```python
from build123d import *

# Parameters (mm, degrees)
SKETCH1_W               = 250
SKETCH1_H               = 50
BOSS_EXTRUDE1_DEPTH     = 55
CUT_EXTRUDE2_DEPTH      = 146.430395722
CUT_EXTRUDE2_DEPTH_BACK = 146.430395722
SKETCH4_OUTSIDE_W       = 304.164
SKETCH4_OUTSIDE_H       = 109.164
FILLET2_R               = 2
CUT_EXTRUDE3_DEPTH      = 143.762915509
CUT_EXTRUDE3_DEPTH_BACK = 143.762915509
SKETCH7_R               = 2.5
SKETCH12_W              = 86.46924187
SKETCH12_H              = 64.710234819
CUT_EXTRUDE7_DEPTH      = 10
CUT_EXTRUDE8_DEPTH      = 10
SKETCH14_R              = 2.5
BOSS_EXTRUDE2_DEPTH     = 30
SKETCH16_W              = 96.26246385
SKETCH16_H              = 15
CUT_EXTRUDE9_DEPTH      = 50
FILLET3_R               = 4.2
FILLET4_R               = 23


with BuildPart() as part:
    # Sketch1 → Boss-Extrude1 (new body)
    with BuildSketch(Plane(origin=(0, 0, 0), x_dir=(1, 0, 0), z_dir=(0, 1, 0))):
        Rectangle(SKETCH1_W, SKETCH1_H)
    extrude(amount=BOSS_EXTRUDE1_DEPTH)

    # Sketch4 outside → Cut-Extrude2 (cut, two sides: drawn at the far end of the back side and taken through both)
    with BuildSketch(Plane.XY.offset(25).offset(-CUT_EXTRUDE2_DEPTH_BACK)):
        with Locations((0, 27.5)):
            Rectangle(SKETCH4_OUTSIDE_W, SKETCH4_OUTSIDE_H)
        with BuildLine():
            Line((-72.5, 42.5), (-72.5, 12.5))
            ThreePointArc((-72.5, 12.5), (16.389156704, 14.940062989), (105, 7.5))
            ThreePointArc((105, 7.5), (125, 27.5), (105, 47.5))
            ThreePointArc((105, 47.5), (16.389156704, 40.059937011), (-72.5, 42.5))
        make_face(mode=Mode.SUBTRACT)
    extrude(amount=CUT_EXTRUDE2_DEPTH + CUT_EXTRUDE2_DEPTH_BACK, mode=Mode.SUBTRACT)

    # Fillet2
    fillet2_edges = [part.edges().sort_by_distance(p)[0] for p in [
        (16.389156704, 14.940062989, 25),
        (16.389156704, 40.059937011, 25),
        (16.389156704, 40.059937011, -25),
        (16.389156704, 14.940062989, -25),
    ]]
    fillet(fillet2_edges, radius=FILLET2_R)

    # Sketch7 → Cut-Extrude3 (cut, two sides: drawn at the far end of the back side and taken through both)
    with BuildSketch(Plane.XY.offset(25).offset(-CUT_EXTRUDE3_DEPTH_BACK)):
        with Locations((105, 27.5)):
            Circle(SKETCH7_R)
    extrude(amount=CUT_EXTRUDE3_DEPTH + CUT_EXTRUDE3_DEPTH_BACK, mode=Mode.SUBTRACT)

    # Sketch12 → Cut-Extrude7 (cut)
    with BuildSketch(Plane.XY.offset(25)):
        with Locations((108.234620935, 27.636294559)):
            Rectangle(SKETCH12_W, SKETCH12_H)
    extrude(amount=-CUT_EXTRUDE7_DEPTH, mode=Mode.SUBTRACT)

    # Sketch13 → Cut-Extrude8 (cut)
    with BuildSketch(Plane(origin=(0, 0, -25), x_dir=(-1, 0, 0), z_dir=(0, 0, -1))):
        with BuildLine():
            Line((-65, 42.911811435), (-65, 12.088188565))
            ThreePointArc((-65, 12.088188565), (-85.028868782, 10.045773403), (-105, 7.5))
            ThreePointArc((-105, 7.5), (-125, 27.5), (-105, 47.5))
            ThreePointArc((-105, 47.5), (-85.028868782, 44.954226597), (-65, 42.911811435))
        make_face()
    extrude(amount=-CUT_EXTRUDE8_DEPTH, mode=Mode.SUBTRACT)

    # Sketch14 → Boss-Extrude2 (add)
    # profile 1 of 2: a face of its own
    with BuildSketch(Plane(origin=(0, 42.5, 0), x_dir=(0, 0, 1), z_dir=(0, -1, 0))):
        with BuildLine():
            Line((-8.002367609, 72.5), (-12.669393759, 94.084995944))
            ThreePointArc((-12.669393759, 94.084995944), (-21.584995944, 99.830606241), (-27.330606241, 90.915004056))
            Line((-27.330606241, 90.915004056), (-23.348983742, 72.5))
            Line((-23.348983742, 72.5), (-8.002367609, 72.5))
        make_face()
        with Locations(Location((-20, 92.5, 0), (0, 0, 180))):
            Circle(SKETCH14_R, mode=Mode.SUBTRACT)
    # profile 2 of 2: a face of its own
    with BuildSketch(Plane(origin=(0, 42.5, 0), x_dir=(0, 0, 1), z_dir=(0, -1, 0))):
        with BuildLine():
            Line((27.330606241, 90.915004056), (23.348983742, 72.5))
            Line((23.348983742, 72.5), (8.002367609, 72.5))
            Line((8.002367609, 72.5), (12.669393759, 94.084995944))
            ThreePointArc((12.669393759, 94.084995944), (21.584995944, 99.830606241), (27.330606241, 90.915004056))
        make_face()
        with Locations((20, 92.5)):
            Circle(SKETCH14_R, mode=Mode.SUBTRACT)
    extrude(amount=BOSS_EXTRUDE2_DEPTH)

    # Sketch16 → Cut-Extrude9 (cut)
    with BuildSketch(Plane.ZY.offset(72.5)):
        with Locations((4.383084191, 27.5)):
            Rectangle(SKETCH16_W, SKETCH16_H)
    extrude(amount=CUT_EXTRUDE9_DEPTH, mode=Mode.SUBTRACT)

    # Fillet3
    fillet3_edges = [part.edges().sort_by_distance(p)[0] for p in [
        (-72.5, 16.25, -8.002367609),
        (-72.5, 16.25, 8.002367609),
        (-72.5, 38.75, 8.002367609),
        (-72.5, 38.75, -8.002367609),
    ]]
    fillet(fillet3_edges, radius=FILLET3_R)

    # Fillet4
    # the kernel refuses this fillet: 23 mm, written as the material it adds along each edge
    with BuildSketch(Plane(origin=(-72.5, 42.030514973, -23.348983742), x_dir=(0, 0, -1), z_dir=(0, -1, 0))) as fillet4_piece_1_section:
        with BuildLine():
            CenterArc((24.342833905, -3.752520734), FILLET4_R, 170.610040363, 21.590428365)
            Line((1.8623081, -8.613174962), (0, 0))
            Line((0, 0), (1.651016258, 0))
        make_face()
    fillet4_piece_1 = extrude(amount=51.530241063, mode=Mode.PRIVATE)
    fillet4_piece_1 = split(fillet4_piece_1, bisect_by=Plane(origin=(-72.5, 35, -23.348983742), z_dir=(0, 1, 0)), keep=Keep.TOP, mode=Mode.PRIVATE)
    add(fillet4_piece_1)
    with BuildSketch(Plane(origin=(-72.5, 20, -23.348983742), x_dir=(0, 0, -1), z_dir=(0, -1, 0))) as fillet4_piece_2_section:
        with BuildLine():
            CenterArc((24.342833905, -3.752520734), FILLET4_R, 170.610040363, 21.590428365)
            Line((1.8623081, -8.613174962), (0, 0))
            Line((0, 0), (1.651016258, 0))
        make_face()
    fillet4_piece_2 = extrude(amount=29.49972609, mode=Mode.PRIVATE)
    fillet4_piece_2 = split(fillet4_piece_2, bisect_by=Plane(origin=(-72.5, 12.5, -23.348983742), z_dir=(0, 1, 0)), keep=Keep.TOP, mode=Mode.PRIVATE)
    add(fillet4_piece_2)
    with BuildSketch(Plane(origin=(-72.5, 64.49972609, -23.348983742), x_dir=(0, 0, -1), z_dir=(0, -1, 0))) as fillet4_piece_3_section:
        with BuildLine():
            CenterArc((24.342833905, -3.752520734), FILLET4_R, 170.610040363, 21.590428365)
            Line((1.8623081, -8.613174962), (0, 0))
            Line((0, 0), (1.651016258, 0))
        make_face()
    fillet4_piece_3 = extrude(amount=29.49972609, mode=Mode.PRIVATE)
    fillet4_piece_3 = split(fillet4_piece_3, bisect_by=Plane(origin=(-72.5, 42.5, -23.348983742), z_dir=(0, -1, 0)), keep=Keep.TOP, mode=Mode.PRIVATE)
    add(fillet4_piece_3)
    with BuildSketch(Plane(origin=(-72.5, 64.49972609, -23.348983742), x_dir=(0, 0, -1), z_dir=(0, -1, 0))) as fillet4_piece_4_section:
        with BuildLine():
            CenterArc((24.342833905, -3.752520734), FILLET4_R, 170.610040363, 21.590428365)
            Line((1.8623081, -8.613174962), (0, 0))
            Line((0, 0), (1.651016258, 0))
        make_face()
    fillet4_piece_4 = extrude(amount=51.530241063, mode=Mode.PRIVATE)
    fillet4_piece_4 = split(fillet4_piece_4, bisect_by=Plane(origin=(-72.5, 20, -23.348983742), z_dir=(0, -1, 0)), keep=Keep.TOP, mode=Mode.PRIVATE)
    add(fillet4_piece_4)
    with BuildSketch(Plane(origin=(-72.5, 42.030514973, 23.348983742), x_dir=(0, 0, 1), z_dir=(0, -1, 0))) as fillet4_piece_5_section:
        with BuildLine():
            CenterArc((24.342833905, 3.752520734), FILLET4_R, 167.799531273, 21.590428365)
            Line((1.8623081, 8.613174962), (0, 0))
            Line((0, 0), (1.651016258, 0))
        make_face()
    fillet4_piece_5 = extrude(amount=51.530241063, mode=Mode.PRIVATE)
    fillet4_piece_5 = split(fillet4_piece_5, bisect_by=Plane(origin=(-72.5, 35, 23.348983742), z_dir=(0, 1, 0)), keep=Keep.TOP, mode=Mode.PRIVATE)
    add(fillet4_piece_5)
    with BuildSketch(Plane(origin=(-72.5, 20, 23.348983742), x_dir=(0, 0, 1), z_dir=(0, -1, 0))) as fillet4_piece_6_section:
        with BuildLine():
            CenterArc((24.342833905, 3.752520734), FILLET4_R, 167.799531273, 21.590428365)
            Line((1.8623081, 8.613174962), (0, 0))
            Line((0, 0), (1.651016258, 0))
        make_face()
    fillet4_piece_6 = extrude(amount=29.49972609, mode=Mode.PRIVATE)
    fillet4_piece_6 = split(fillet4_piece_6, bisect_by=Plane(origin=(-72.5, 12.5, 23.348983742), z_dir=(0, 1, 0)), keep=Keep.TOP, mode=Mode.PRIVATE)
    add(fillet4_piece_6)
    with BuildSketch(Plane(origin=(-72.5, 64.49972609, 23.348983742), x_dir=(0, 0, 1), z_dir=(0, -1, 0))) as fillet4_piece_7_section:
        with BuildLine():
            CenterArc((24.342833905, 3.752520734), FILLET4_R, 167.799531273, 21.590428365)
            Line((1.8623081, 8.613174962), (0, 0))
            Line((0, 0), (1.651016258, 0))
        make_face()
    fillet4_piece_7 = extrude(amount=29.49972609, mode=Mode.PRIVATE)
    fillet4_piece_7 = split(fillet4_piece_7, bisect_by=Plane(origin=(-72.5, 42.5, 23.348983742), z_dir=(0, -1, 0)), keep=Keep.TOP, mode=Mode.PRIVATE)
    add(fillet4_piece_7)
    with BuildSketch(Plane(origin=(-72.5, 64.49972609, 23.348983742), x_dir=(0, 0, 1), z_dir=(0, -1, 0))) as fillet4_piece_8_section:
        with BuildLine():
            CenterArc((24.342833905, 3.752520734), FILLET4_R, 167.799531273, 21.590428365)
            Line((1.8623081, 8.613174962), (0, 0))
            Line((0, 0), (1.651016258, 0))
        make_face()
    fillet4_piece_8 = extrude(amount=51.530241063, mode=Mode.PRIVATE)
    fillet4_piece_8 = split(fillet4_piece_8, bisect_by=Plane(origin=(-72.5, 20, 23.348983742), z_dir=(0, -1, 0)), keep=Keep.TOP, mode=Mode.PRIVATE)
    add(fillet4_piece_8)


solid = part.part
```
For this review, take the finished solid that the model builds, in its own axes (mm). A direction names the side the tool comes from. Coordinates: 2 decimals unless noted, no trailing zeros. Loops run counter-clockwise (first coordinate to the right, second up) from the corner with the lowest first, then second, coordinate; pieces in that order, holes last.
1. For faces 5 (the flat face through (-86, 42.5, 19)), 6 (the flat face through (-84.821, 38.802, 10.666)), 7 (the flat face through (-5, 27, -25)), list the 3-axis set-ups (+Z, -Z, +X, -X, +Y, -Y) from which the entire face can be reached by the end or side of a thin tool; tool diameter is ignored.
2. Add section B-B, the plane y = 27.5. Give the boundary of the cut face in (x, z).
3. For line 1 (X direction, y = 15.75, z = -20); line 2 (Z direction, x = -92, y = 18); line 3 (Y direction, x = 105, z = -8), list the stretches that pass through material, from the lowest coordinate up.
4. Mouldability with a two-part tool opening along Y and no side actions: class faces 1 (the flat face through (-72.5, 28, 0)), 2 (the flat face through (-86, 35, -19)), 3 (the flat face through (-86.083, 16.303, 26.286)), 4 (the flat face through (-86, 12.5, -19)) as +Y half, -Y half, draft (parallel to the pull), parting line (faces both ways), or undercut.
5. Insertion check: P1, Ø8, axis at y = 22, z = 21.5, coming from the +X side; P2, Ø4, axis at x = -35.5, y = 36.5, coming from the +Z side; P3, Ø12, axis at x = 69, z = 1.5, coming from the +Y side. Each pin has a flat end and moves straight along its axis. Give the tip position at first contact, or say it passes through.
6. Add section A-A, the plane z = -20. Give the boundary of the cut face in (x, y), then the cut area to 3 significant figures.
Result:
1. face 5: +Z, -Z, -X, +Y
1. face 6: -X, +Y, -Y
1. face 7: -Z, +X, +Y, -Y
2. outline: (-72.5, -25) - (65, -25) - (65, -15) - (102.5, -15) - (102.5, 15) - (65, 15) - (65, 25) - (-72.5, 25) - close; (107.5, -15) - (125, -15) - (125, 15) - (107.5, 15) - close
3. line 1: x = -100 to -95, -90 to 65
3. line 2: z = -27.48 to -22.45, -17.55 to -12.22, 12.22 to 17.55, 22.45 to 27.48
3. line 3: y = 7.5 to 25, 30 to 47.5
4. face 1: undercut
4. face 2: undercut
4. face 3: draft
4. face 4: -Y half
5. P1: stops at x = 65
5. P2: stops at z = 25
5. P3: stops at y = 43.87
6. outline: (-100, 12.5) - (-95, 12.5) - (-95, 20) - (-100, 20) - close; (-100, 35) - (-95, 35) - (-95, 42.5) - (-100, 42.5) - close; (-90, 12.5) - (-72.5, 12.5) arc R800 cw to (65, 12.09) - (65, 42.91) arc R800 cw to (-72.5, 42.5) - (-90, 42.5) - (-90, 35) - (-72.5, 35) - (-72.5, 20) - (-90, 20) - close
6. area: 3,980 mm2
